Build history of the part. All positions in model axes, mm. A direction names the side the tool comes from. Give positions to 0.01 mm unless a question says otherwise; leave off trailing zeros. Write each loop counter-clockwise with the first axis right and the second up, starting at its lowest first coordinate (ties: lowest second). Pieces come first, ordered by that corner, then holes. Notation, with made-up numbers: (0.25, 87) -> (59.25, 87) arc R28 cw to (59.25, 125) -> close; hole circle Ø8 at (-2, 38.5). An arc over 180 degrees is marked (long way). Write item = value, one per line. Start each with the question number.
Q1. Mould opens along Y. For faces 4 (the face through (1, 123, -16)), 5 (the face through (2, 100, -6)), 6 (the face through (1, 51, 0)), 7 (the face through (2, 41, -12)) say: pulls with the +Y half, pulls with the -Y half, needs draft (parallel to the pull), parting line crosses it, or undercut.
Q2. Wall check: line 1 (Y direction, x = 1.8, z = -3). Give the ranges that are in metal, low to high.
Q3. Saw through at B-B, the plane x = 0.6. List the corners of the cut face in (y, z).
Q4. Drop flat-ended pins along their axis: P1, Ø0.9, axis at x = 1.5, y = 121.5, coming from the +Z side; P2, Ø0.9, axis at x = 2, z = -7, coming from the +Y side; P3, Ø1.5, axis at x = 2, z = -5.5, coming from the -Y side. Give the stop position or say it passes through.
Q5. Tool access for faces 1 (the face through (1, 31, 0)), 2 (the face through (2, 1, -12)), 3 (the face through (2, 101, -12)): list every direction of +Z, -Z, +X, -X, +Y, -Y with a clear straight run to the whole face (end or side of a thin tool).
Q6. Saw through at C-C, the plane y = 61. List the corners of the cut face in (x, z), then the cut area to 3 significant figures.
Q7. Saw through at A-A, the plane z = -4. List the corners of the cut face in (x, y).
from build123d import *

# Parameters (mm, degrees)
SKETCH1_W           = 20
SKETCH1_H           = 123
BOSS_EXTRUDE1_DEPTH = 3
SKETCH2_W           = 12
SKETCH2_H           = 3
CUT_EXTRUDE1_DEPTH  = 125.651514231
LPATTERN1_COUNT     = 7
LPATTERN1_PITCH     = 20


with BuildPart() as part:
    # Sketch1 → Boss-Extrude1 (new body)
    with BuildSketch(Plane(origin=(0, 0, 0), x_dir=(0, 0, -1), z_dir=(1, 0, 0))):
        with Locations((10, 61.5)):
            Rectangle(SKETCH1_W, SKETCH1_H)
    extrude(amount=BOSS_EXTRUDE1_DEPTH)

    # Sketch2 → Cut-Extrude1 (cut, through all)
    with BuildSketch(Plane(origin=(3, 0, 0), x_dir=(0, 0, -1), z_dir=(1, 0, 0))):
        with Locations((6, 1.5)):
            Rectangle(SKETCH2_W, SKETCH2_H)
    cut_extrude1 = extrude(amount=-CUT_EXTRUDE1_DEPTH, mode=Mode.SUBTRACT)

    # LPattern1: Cut-Extrude1 ×7
    with Locations(*[(0, i * LPATTERN1_PITCH, 0) for i in range(1, LPATTERN1_COUNT)]):
        add(cut_extrude1, mode=Mode.SUBTRACT)


solid = part.part
Report:
q1.face_4 = pulls with the +Y half
q1.face_5 = undercut
q1.face_6 = needs draft
q1.face_7 = undercut
q2.line_1 = 3 to 20, 23 to 40, 43 to 60, 63 to 80, 83 to 100, 103 to 120
q3.outline = (0, -20) -> (123, -20) -> (123, -12) -> (120, -12) -> (120, 0) -> (103, 0) -> (103, -12) -> (100, -12) -> (100, 0) -> (83, 0) -> (83, -12) -> (80, -12) -> (80, 0) -> (63, 0) -> (63, -12) -> (60, -12) -> (60, 0) -> (43, 0) -> (43, -12) -> (40, -12) -> (40, 0) -> (23, 0) -> (23, -12) -> (20, -12) -> (20, 0) -> (3, 0) -> (3, -12) -> (0, -12) -> close
q4.P1 = -12
q4.P2 = 120
q4.P3 = 3
q5.face_1 = +Z, +X, -X, +Y, -Y
q5.face_2 = +Z, +X, -X, -Y
q5.face_3 = +Z, +X, -X
q6.outline = (0, -20) -> (3, -20) -> (3, -12) -> (0, -12) -> close
q6.area = 24.0 mm2
q7.outline = (0, 3) -> (3, 3) -> (3, 20) -> (0, 20) -> close; (0, 23) -> (3, 23) -> (3, 40) -> (0, 40) -> close; (0, 43) -> (3, 43) -> (3, 60) -> (0, 60) -> close; (0, 63) -> (3, 63) -> (3, 80) -> (0, 80) -> close; (0, 83) -> (3, 83) -> (3, 100) -> (0, 100) -> close; (0, 103) -> (3, 103) -> (3, 120) -> (0, 120) -> close
